```python
from build123d import *

# Parameters (mm, degrees)
BOSS_EXTRUDE1_DEPTH = 80


with BuildPart() as part:
    # Sketch1 → Boss-Extrude1 (new body)
    with BuildSketch(Plane.XY):
        with BuildLine():
            Line((0, 0), (0, -6))
            Line((0, -6), (-1, -6))
            ThreePointArc((-1, -6), (-2.414213562, -5.414213562), (-3, -4))
            Line((-3, -4), (-3, 0))
            ThreePointArc((-3, 0), (-2.414213562, 1.414213562), (-1, 2))
            Line((-1, 2), (4, 2))
            Line((4, 2), (4, 0))
            Line((4, 0), (0, 0))
        make_face()
    extrude(amount=BOSS_EXTRUDE1_DEPTH)


solid = part.part
```
Here's how the part is built. I have some questions about the finished solid (model axes, mm). A direction names the side the tool comes from. Give positions to 0.01 mm unless a question says otherwise; leave off trailing zeros. Loops run counter-clockwise (first coordinate to the right, second up) from the corner with the lowest first, then second, coordinate; pieces in that order, holes last. Notation, with made-up numbers: M -2,46.5 L 52,46.5 A9 cw 52,63.5 Z; hole C -6.75,35 d4. An arc over 180 degrees is marked long. Put each result on its own line as item: value. Start each with the question number.
(1) I want a section at C-C on y = -3.25. Please give me the cut outline in (x, z), then the cut area to 3 significant figures.
(2) I need wall thicknesses on line 1 along X through (y, z) = (-4, 4); line 2 along Y through (x, z) = (-1.25, 53); line 3 along Y through (x, z) = (3.75, 41). Which ranges of each line are inside material? Lowest first, please. Write a range as [from, to].
(3) For faces 1 (the flat face through (1, 2, 39)), 2 (the flat face through (0, -3, 39)), which set-ups out of +Z, -Z, +X, -X, +Y, -Y let a thin tool reach every point of the face, with its end or its side?
(4) I want a section at B-B on x = 2.75. Please give me the cut outline in (y, z), then the cut area to 3 significant figures.
(5) I want a section at A-A on z = 58.5. Please give me the cut outline in (x, y), then the cut area to 3 significant figures.
(6) Will this pin go through, and if not, where does the flat tip stop? pin 1 Ø1.2 at (x, z) = (1, 36.5) entering from -Y.
Answer block:
1. outline: M -3,0 L 0,0 L 0,80 L -3,80 Z
1. area: 240 mm^2
2. line 1: [-3, 0]
2. line 2: [-5.98, 1.98]
2. line 3: [0, 2]
3. face 1: +Z, -Z, +X, -X, +Y
3. face 2: +Z, -Z, +X, -Y
4. outline: M 0,0 L 2,0 L 2,80 L 0,80 Z
4. area: 160 mm^2
5. outline: M -3,-4 A2 ccw -1,-6 L 0,-6 L 0,0 L 4,0 L 4,2 L -1,2 A2 ccw -3,0 Z
5. area: 30.3 mm^2
6. pin 1: y = 0
